Design review of the part built by this model. Coordinates are the model's own, in mm. A direction names the side the tool comes from. Give positions to 0.01 mm unless a question says otherwise; leave off trailing zeros. Write each loop counter-clockwise with the first axis right and the second up, starting at its lowest first coordinate (ties: lowest second). Pieces come first, ordered by that corner, then holes. Notation, with made-up numbers: M 13,24 L 31,24 A30 ccw 31,46 Z; hole C 20,85 d1. An arc over 180 degrees is marked long. Answer in a Markdown table with one row per item.
```python
from build123d import *

# Parameters (mm, degrees)
M1X0_25_1_D         = 0.75
CUT_EXTRUDE_START   = -2
CUT_EXTRUDE_1_DEPTH = 2
FILLET_1_R          = 1.5


# Read off the part's stored shape, not the designer's step: ｶｯﾄ - 押し出し1
with BuildPart() as part:
    # ｽｹｯﾁ1 → 回転1 (revolve)
    with BuildSketch(Plane(origin=(0, 0, 0), x_dir=(0, 0, -1), z_dir=(1, 0, 0)), mode=Mode.PRIVATE) as revolve_1_sk:
        Polygon((0, 4), (2.9, 4), (2.9, 17.5), (0.9, 17.5), (0.9, 5), (0, 5), align=None)
    revolve(revolve_1_sk.sketch.rotate(Axis((0, 0, 0), (0, 0, -1)), 90), axis=Axis((0, 0, 0), (0, 0, -1)))

    # M1x0.25 ねじ穴1 (through all)
    with Locations(Plane.XY.offset(-0.9)):
        with Locations((9.999999803, 0), (-5, 8.660254038), (-5.000000098, -8.660253981)):
            Hole(M1X0_25_1_D / 2)

    # ｶｯﾄ - 押し出し1 outline → ｶｯﾄ - 押し出し1 (cut)
    with BuildSketch(Plane.XY.offset(-0.9).offset(CUT_EXTRUDE_START)):
        with BuildLine():
            ThreePointArc((-4.91198547, -3.445634737), (-6, 0), (-4.91198547, 3.445634737))
            ThreePointArc((-4.91198547, 3.445634737), (-4.731685773, 4.823475601), (-5.759987903, 5.758113582))
            ThreePointArc((-5.759987903, 5.758113582), (-6.819518607, 6.275017773), (-7.598076211, 7.160254038))
            Line((-7.598076211, 7.160254038), (-9.179299502, 9.899013115))
            ThreePointArc((-9.179299502, 9.899013115), (-13.5, 8.7e-08), (-9.17929963, -9.899012996))
            Line((-9.17929963, -9.899012996), (-7.59807631, -7.160253868))
            ThreePointArc((-7.59807631, -7.160253868), (-6.819518691, -6.275017592), (-5.759987933, -5.758113538))
            ThreePointArc((-5.759987933, -5.758113538), (-4.731685776, -4.823475609), (-4.91198547, -3.445634737))
        make_face()
        with BuildLine():
            ThreePointArc((5.43999995, -2.531086831), (3, -5.196152423), (-0.52801448, -5.976721569))
            ThreePointArc((-0.52801448, -5.976721569), (-1.811409498, -6.509497859), (-2.106678705, -7.86735258))
            ThreePointArc((-2.106678705, -7.86735258), (-2.024565604, -9.043385134), (-2.401923887, -10.160253868))
            Line((-2.401923887, -10.160253868), (-3.983147246, -12.899013064))
            ThreePointArc((-3.983147246, -12.899013064), (6.749999924, -11.691342995), (13.162446581, -3))
            Line((13.162446581, -3), (9.999999803, -3))
            ThreePointArc((9.999999803, -3), (8.84408395, -2.768367486), (7.866666559, -2.109239026))
            ThreePointArc((7.866666559, -2.109239026), (6.543095269, -1.686022286), (5.43999995, -2.531086831))
        make_face()
        with BuildLine():
            ThreePointArc((-0.52801448, 5.976721569), (3, 5.196152423), (5.43999995, 2.531086831))
            ThreePointArc((5.43999995, 2.531086831), (6.543095269, 1.686022286), (7.866666559, 2.109239026))
            ThreePointArc((7.866666559, 2.109239026), (8.84408395, 2.768367486), (9.999999803, 3))
            Line((9.999999803, 3), (13.162446581, 3))
            ThreePointArc((13.162446581, 3), (6.75, 11.691342951), (-3.983147079, 12.899013115))
            Line((-3.983147079, 12.899013115), (-2.401923789, 10.160254038))
            ThreePointArc((-2.401923789, 10.160254038), (-2.024565497, 9.043385242), (-2.106678823, 7.867352678))
            ThreePointArc((-2.106678823, 7.867352678), (-1.811409518, 6.509497883), (-0.52801448, 5.976721569))
        make_face()
    extrude(amount=CUT_EXTRUDE_1_DEPTH, mode=Mode.SUBTRACT)

    # ﾌｨﾚｯﾄ1
    fillet_1_edges = [part.edges().sort_by_distance(p)[0] for p in [
        (-9.17929963, -9.899012996, -1.9),
        (-9.179299502, 9.899013115, -1.9),
        (-3.983147079, 12.899013115, -1.9),
        (13.162446581, 3, -1.9),
        (13.162446581, -3, -1.9),
        (-3.983147246, -12.899013064, -1.9),
    ]]
    fillet(fillet_1_edges, radius=FILLET_1_R)


solid = part.part
```
1) Insertion check: P1, Ø1, axis at x = -13.5, z = -1, coming from the +Y side; P2, Ø1.2, axis at x = 10.5, z = -2, coming from the +Y side; P3, Ø1.5, axis at x = 12.5, z = -1, coming from the -Y side. Each pin has a flat end and moves straight along its axis. Give the tip position at first contact, or say it passes through.
Geometry says:
| item | result |
|---|---|
| P1 | y = 11.72 |
| P2 | y = 14.43 |
| P3 | y = -12.97 |
2) Add section A-A (x = 0). Write out the cut boundary in (y, z).
Geometry says:
| item | result |
|---|---|
| outline | M -17.5,-2.9 L -13.5,-2.9 L -13.5,-0.9 L -17.5,-0.9 Z; M -6,-2.9 L -4,-2.9 L -4,0 L -5,0 L -5,-0.9 L -6,-0.9 Z; M 4,-2.9 L 6,-2.9 L 6,-0.9 L 5,-0.9 L 5,0 L 4,0 Z; M 13.5,-2.9 L 17.5,-2.9 L 17.5,-0.9 L 13.5,-0.9 Z |
3) Add section C-C (x = -6.5). Write out the cut boundary in (y, z).
Geometry says:
| item | result |
|---|---|
| outline | M -16.25,-2.9 L -6.06,-2.9 L -6.06,-0.9 L -16.25,-0.9 Z; M 6.06,-2.9 L 16.25,-2.9 L 16.25,-0.9 L 6.06,-0.9 Z |
4) The part is to be moulded in two halves that separate along Y. For faces 3 (the face through (-4, 4, -2.9)), 4 (the face through (-9.38, -8.88, -1.89)), 5 (the face through (-6.833, -6.285, -1.914)), 6 (the face through (-4.995, -0.22, -0.444)), say which applies: released by +Y, released by -Y, zero draft, split by the parting line, or undercut.
Geometry says:
| item | result |
|---|---|
| face 3 | zero draft |
| face 4 | undercut |
| face 5 | undercut |
| face 6 | split by the parting line |
5) Add section D-D (y = -1). Write out the cut boundary in (x, z).
Geometry says:
| item | result |
|---|---|
| outline | M -17.47,-2.9 L -13.46,-2.9 L -13.46,-0.9 L -17.47,-0.9 Z; M -5.92,-2.9 L -3.87,-2.9 L -3.87,0 L -4.9,0 L -4.9,-0.9 L -5.92,-0.9 Z; M 3.87,-2.9 L 17.47,-2.9 L 17.47,-0.9 L 4.9,-0.9 L 4.9,0 L 3.87,0 Z |
6) For faces 1 (the face through (6.52, 1.69, -1.91)), 2 (the face through (4, 4, -0.9)), list the 3-axis set-ups (+Z, -Z, +X, -X, +Y, -Y) from which the entire face can be reached by the end or side of a thin tool; tool diameter is ignored.
Geometry says:
| item | result |
|---|---|
| face 1 | +Z, -Z |
| face 2 | +Z |
7) Add section B-B (y = -9.5). Write out the cut boundary in (x, z), and give its area (3 significant figures).
Geometry says:
| item | result |
|---|---|
| outline | M -14.7,-2.9 L -2.12,-2.9 L -2.12,-0.9 L -14.7,-0.9 Z; M 9.59,-2.9 L 14.7,-2.9 L 14.7,-0.9 L 9.59,-0.9 Z |
| area | 35.4 mm^2 |
8) To check wall thickness, follow probe 1 along Y at (x, z) = (0, -2.15); probe 2 along Y at (x, z) = (-5, -2.2); probe 3 along Y at (x, z) = (10, -2.1) (3 decimals). State the ranges of each line that lie inside material, in increasing order. Write a range as [from, to].
Geometry says:
| item | result |
|---|---|
| probe 1 | [-17.5, -13.5], [-6, -4], [4, 6], [13.5, 17.5] |
| probe 2 | [-16.77, -9.04], [-8.29, -5.28], [-3.32, 3.32], [5.28, 8.29], [9.04, 16.77] |
| probe 3 | [-14.361, -9.069], [-3, -0.375], [0.375, 3], [9.069, 14.361] |
